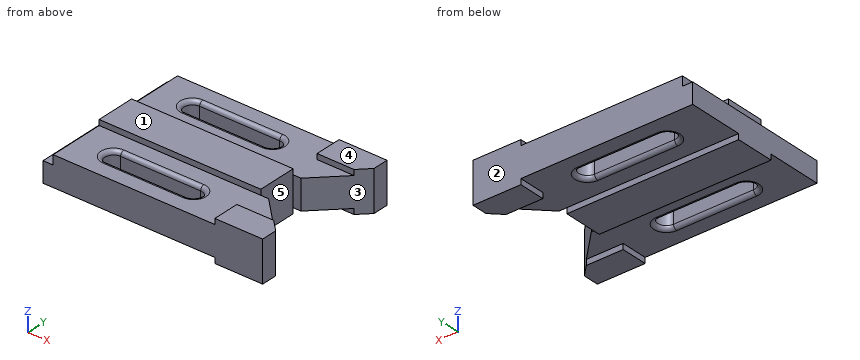
```python
from build123d import *

# Parameters (mm, degrees)
SKETCH1_W           = 109.5
SKETCH1_H           = 25
BOSS_EXTRUDE3_DEPTH = 9.5
BOSS_EXTRUDE4_DEPTH = 3.5
BOSS_EXTRUDE5_DEPTH = 3.5
BOSS_EXTRUDE6_DEPTH = 3.5
BOSS_EXTRUDE7_DEPTH = 3.5
SKETCH13_W          = 109.5
SKETCH13_H          = 25
BOSS_EXTRUDE8_DEPTH = 3.5
SKETCH14_W          = 109.5
SKETCH14_H          = 25
BOSS_EXTRUDE9_DEPTH = 3.5
CUT_EXTRUDE1_DEPTH  = 44
FILLET1_R           = 2.5
SKETCH16_W          = 6.5
SKETCH16_H          = 96
CUT_EXTRUDE2_DEPTH  = 11.5


with BuildPart() as part:
    # Sketch1 → Boss-Extrude3 (new, symmetric)
    # profile 1 of 7: a face of its own
    with BuildSketch(Plane.XY):
        Polygon((104.5, 31), (104.5, 48), (0, 48), (0, 12.5), (109.5, 12.5), (114.5, 12.5), (133, 31), align=None)
        with BuildLine():
            ThreePointArc((30.5, 25), (25, 30.5), (30.5, 36))
            Line((30.5, 36), (81.5, 36))
            ThreePointArc((81.5, 36), (87, 30.5), (81.5, 25))
            Line((81.5, 25), (30.5, 25))
        make_face(mode=Mode.SUBTRACT)
    # profile 2 of 7: a face of its own
    with BuildSketch(Plane.XY):
        with BuildLine():
            Line((30.5, 25), (81.5, 25))
            ThreePointArc((81.5, 25), (87, 30.5), (81.5, 36))
            Line((81.5, 36), (30.5, 36))
            ThreePointArc((30.5, 36), (25, 30.5), (30.5, 25))
        make_face()
    # profile 3 of 7: a face of its own
    with BuildSketch(Plane.XY):
        Polygon((140, 38), (140, 48), (104.5, 48), (104.5, 31), (133, 31), align=None)
    # profile 4 of 7: a face of its own
    with BuildSketch(Plane.XY):
        with Locations((54.75, 0)):
            Rectangle(SKETCH1_W, SKETCH1_H)
    # profile 5 of 7: a face of its own
    with BuildSketch(Plane.XY):
        Polygon((104.5, -31), (104.5, -48), (140, -48), (140, -38), (133, -31), align=None)
    # profile 6 of 7: a face of its own
    with BuildSketch(Plane.XY):
        Polygon((109.5, -12.5), (0, -12.5), (0, -48), (104.5, -48), (104.5, -31), (133, -31), (114.5, -12.5), align=None)
        with BuildLine():
            Line((81.5, -36), (30.5, -36))
            ThreePointArc((30.5, -36), (25, -30.5), (30.5, -25))
            Line((30.5, -25), (81.5, -25))
            ThreePointArc((81.5, -25), (87, -30.5), (81.5, -36))
        make_face(mode=Mode.SUBTRACT)
    # profile 7 of 7: a face of its own
    with BuildSketch(Plane.XY):
        with BuildLine():
            ThreePointArc((81.5, -25), (87, -30.5), (81.5, -36))
            Line((81.5, -36), (30.5, -36))
            ThreePointArc((30.5, -36), (25, -30.5), (30.5, -25))
            Line((30.5, -25), (81.5, -25))
        make_face()
    extrude(amount=BOSS_EXTRUDE3_DEPTH, both=True)

    # Sketch9 → Boss-Extrude4 (add, symmetric)
    with BuildSketch(Plane.XY.offset(9.5)):
        Polygon((140, 48), (140, 38), (133, 31), (109.5, 31), (109.5, 48), align=None)
    extrude(amount=BOSS_EXTRUDE4_DEPTH, both=True)

    # Sketch10 → Boss-Extrude5 (add, symmetric)
    with BuildSketch(Plane(origin=(0, 0, -9.5), x_dir=(-1, 0, 0), z_dir=(0, 0, -1))):
        Polygon((-109.5, 48), (-140, 48), (-140, 38), (-133, 31), (-109.5, 31), align=None)
    extrude(amount=BOSS_EXTRUDE5_DEPTH, both=True)

    # Sketch11 → Boss-Extrude6 (add, symmetric)
    with BuildSketch(Plane.XY.offset(9.5)):
        Polygon((140, -38), (140, -48), (109.5, -48), (109.5, -31), (133, -31), align=None)
    extrude(amount=BOSS_EXTRUDE6_DEPTH, both=True)

    # Sketch12 → Boss-Extrude7 (add, symmetric)
    with BuildSketch(Plane(origin=(0, 0, -9.5), x_dir=(-1, 0, 0), z_dir=(0, 0, -1))):
        Polygon((-140, -48), (-140, -38), (-133, -31), (-109.5, -31), (-109.5, -48), align=None)
    extrude(amount=BOSS_EXTRUDE7_DEPTH, both=True)

    # Sketch13 → Boss-Extrude8 (add, symmetric)
    with BuildSketch(Plane.XY.offset(9.5)):
        with Locations((54.75, 0)):
            Rectangle(SKETCH13_W, SKETCH13_H)
    extrude(amount=BOSS_EXTRUDE8_DEPTH, both=True)

    # Sketch14 → Boss-Extrude9 (add, symmetric)
    with BuildSketch(Plane(origin=(0, 0, -9.5), x_dir=(-1, 0, 0), z_dir=(0, 0, -1))):
        with Locations((-54.75, 0)):
            Rectangle(SKETCH14_W, SKETCH14_H)
    extrude(amount=BOSS_EXTRUDE9_DEPTH, both=True)

    # Sketch15 → Cut-Extrude1 (cut)
    with BuildSketch(Plane.XY.offset(9.5)):
        with BuildLine():
            Line((30.5, 36), (81.5, 36))
            ThreePointArc((81.5, 36), (87, 30.5), (81.5, 25))
            Line((81.5, 25), (30.5, 25))
            ThreePointArc((30.5, 25), (25, 30.5), (30.5, 36))
        make_face()
        with BuildLine():
            Line((30.5, -25), (81.5, -25))
            ThreePointArc((81.5, -25), (87, -30.5), (81.5, -36))
            Line((81.5, -36), (30.5, -36))
            ThreePointArc((30.5, -36), (25, -30.5), (30.5, -25))
        make_face()
    extrude(amount=-CUT_EXTRUDE1_DEPTH, mode=Mode.SUBTRACT)

    # Fillet1
    fillet1_edges = [part.edges().sort_by_distance(p)[0] for p in [
        (25, 30.5, -9.5),
        (56, 36, -9.5),
        (87, 30.5, -9.5),
        (56, 25, -9.5),
        (25, 30.5, 9.5),
        (56, 25, 9.5),
        (87, 30.5, 9.5),
        (56, 36, 9.5),
        (25, -30.5, -9.5),
        (56, -25, -9.5),
        (87, -30.5, -9.5),
        (56, -36, -9.5),
        (25, -30.5, 9.5),
        (56, -36, 9.5),
        (87, -30.5, 9.5),
        (56, -25, 9.5),
    ]]
    fillet(fillet1_edges, radius=FILLET1_R)

    # Sketch16 → Cut-Extrude2 (cut)
    with BuildSketch(Plane.XY.offset(15)):
        with Locations((3.25, 0)):
            Rectangle(SKETCH16_W, SKETCH16_H)
    extrude(amount=-CUT_EXTRUDE2_DEPTH, mode=Mode.SUBTRACT)


solid = part.part
```
Here's how the part is built. I have some questions about the finished solid (model axes, mm). Face numbers are marked on the shaded views. A direction names the side the tool comes from. Give positions to 0.01 mm unless a question says otherwise; leave off trailing zeros. Loops run counter-clockwise (first coordinate to the right, second up) from the corner with the lowest first, then second, coordinate; pieces in that order, holes last. Notation, with made-up numbers: M 36.25,66 L 72.25,66 A13 ccw 72.25,73 Z; hole C 20,85.25 d7. An arc over 180 degrees is marked long. Put each result on its own line as item: value. Start each with the question number.
(1) For the marked faces 4 and 5, which set-ups out of +Z, -Z, +X, -X, +Y, -Y let a thin tool reach every point of the face, with its end or its side?
(2) I want a section at A-A on x = 34. Please give me the cut outline in (y, z).
(3) I need wall thicknesses on line 1 along Y through (x, z) = (66.5, -0.75); line 2 along Y through (x, z) = (131, 11.25); line 3 along Y through (x, z) = (29, -4.75). Which ranges of each line are inside material? Lowest first, please. Write a range as [from, to].
(4) I want a section at C-C on z = -4. Please give me the cut outline in (x, y), then the cut area to 3 significant figures.
(5) If we mould it in two halves opening along Y, with no side actions, what happens to the marked faces 1, 2 and 3? For each: +Y half, -Y half, draft (parallel to the pull), parting line (faces both ways), or undercut.
(6) I want a section at D-D on y = -7. Please give me the cut outline in (x, z), then the cut area to 3 significant figures.
(7) Will these pins go through, and if not, where does the flat tip stop? pin 1 Ø10.5 at (x, y) = (47.5, 22.5) entering from +Z; pin 2 Ø1.5 at (y, z) = (11, -6) entering from +X; pin 3 Ø8 at (y, z) = (25, 3.5) entering from +X.
(8) I want a section at B-B on x = 113. Please give me the cut outline in (y, z).
Answer block:
1. face 4: +Z, +X, -X, +Y, -Y
1. face 5: +Z, -Z, +X
2. outline: M -48,-9.5 L -38.5,-9.5 A2.5 ccw -36,-7 L -36,7 A2.5 ccw -38.5,9.5 L -48,9.5 Z; M -25,-7 A2.5 ccw -22.5,-9.5 L -12.5,-9.5 L -12.5,-13 L 12.5,-13 L 12.5,-9.5 L 22.5,-9.5 A2.5 ccw 25,-7 L 25,7 A2.5 ccw 22.5,9.5 L 12.5,9.5 L 12.5,13 L -12.5,13 L -12.5,9.5 L -22.5,9.5 A2.5 ccw -25,7 Z; M 36,-7 A2.5 ccw 38.5,-9.5 L 48,-9.5 L 48,9.5 L 38.5,9.5 A2.5 ccw 36,7 Z
3. line 1: [-48, -36], [-25, 25], [36, 48]
3. line 2: [-48, -31], [31, 48]
3. line 3: [-48, -35.79], [-25.21, 25.21], [35.79, 48]
4. outline: M 0,-48 L 140,-48 L 140,-38 L 114.5,-12.5 L 109.5,-12.5 L 109.5,12.5 L 114.5,12.5 L 140,38 L 140,48 L 0,48 Z; hole M 30.5,-36 L 81.5,-36 A5.5 ccw 81.5,-25 L 30.5,-25 A5.5 ccw Z; hole M 30.5,25 L 81.5,25 A5.5 ccw 81.5,36 L 30.5,36 A5.5 ccw Z
4. area: 10,700 mm^2
5. face 1: draft
5. face 2: +Y half
5. face 3: undercut
6. outline: M 0,-13 L 109.5,-13 L 109.5,13 L 6.5,13 L 6.5,3.5 L 0,3.5 Z
6. area: 2,790 mm^2
7. pin 1: z = 9.5
7. pin 2: x = 109.5
7. pin 3: x = 131
8. outline: M -48,-13 L -31,-13 L -31,-9.5 L -12.5,-9.5 L -12.5,9.5 L -31,9.5 L -31,13 L -48,13 Z; M 12.5,-9.5 L 31,-9.5 L 31,-13 L 48,-13 L 48,13 L 31,13 L 31,9.5 L 12.5,9.5 Z
